Drawing for the job (mm, zero at the part's lowest x, y, z). A direction names the side the tool comes from. Round coordinates to 2 decimals unless told otherwise and drop trailing zeros. Write each loop counter-clockwise with the first axis right and the second up, starting at its lowest first coordinate (ties: lowest second). Pieces come first, ordered by that corner, then holes. Notation, with made-up numbers: M -7,15 L 2,15 A8 ccw 2,25 Z; hole C 60,19.5 d9. An arc over 180 degrees is marked long. Use a Markdown table: item, result.
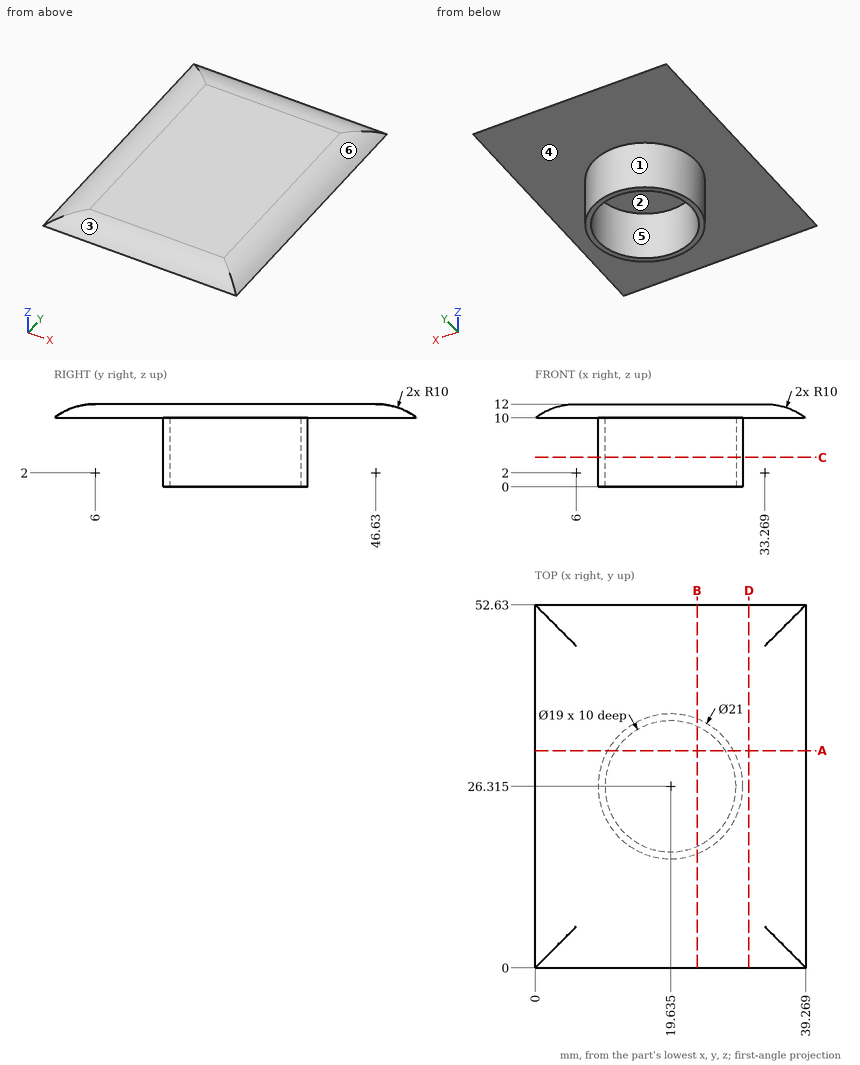
Q1. Which spindle directions (+Z, -Z, +X, -X, +Y, -Y) get a long thin tool onto all of the face, cutting with end or side? Do the marked faces 5 and 6. Say none if no direction does.
Response values:
| item | result |
|---|---|
| face 5 | -Z |
| face 6 | +Z, +X, +Y, -Y |
Q2. Drill centre lines: L1, parallel to X at y = 26, z = 2.25; L2, parallel to Y at x = 21, z = 3.5 (1 decimal); L3, parallel to Z at x = 18, y = 23. Where is each one in solid material? Low to high.
Response values:
| item | result |
|---|---|
| L1 | x = 9.14 to 10.14, 29.13 to 30.13 |
| L2 | y = 15.9 to 16.9, 35.7 to 36.7 |
| L3 | z = 10 to 12 |
Q3. Cut at C-C on z = 4.25. Give the cut face in (x, y) (1 decimal).
Response values:
| item | result |
|---|---|
| outline | C 19.6,26.3 d21; hole C 19.6,26.3 d19 |
Q4. Drop flat-ended pins along their axis: P1, Ø4, axis at y = 23, z = 9, coming from the +X side; P2, Ø11.5, axis at x = 19.63, y = 26.32, coming from the -Z side; P3, Ø1, axis at x = 22, z = 9, coming from the -Y side. Give the stop position or say it passes through.
Response values:
| item | result |
|---|---|
| P1 | stops at x = 39.27 |
| P2 | stops at z = 10 |
| P3 | stops at y = 15.98 |
Q5. Cut at A-A on y = 31.5. Give the cut face in (x, z) (1 decimal).
Response values:
| item | result |
|---|---|
| outline | M 0,10 L 10.5,10 L 10.5,0 L 11.7,0 L 11.7,10 L 27.6,10 L 27.6,0 L 28.8,0 L 28.8,10 L 39.3,10 A10 ccw 33.3,12 L 6,12 A10 ccw Z |
Q6. Cut at D-D on x = 31. Give the cut face in (y, z).
Response values:
| item | result |
|---|---|
| outline | M 0,10 L 52.63,10 A10 ccw 46.63,12 L 6,12 A10 ccw Z |
Q7. Cut at B-B on x = 23.5. Give the cut face in (y, z).
Response values:
| item | result |
|---|---|
| outline | M 0,10 L 16.55,10 L 16.55,0 L 17.64,0 L 17.64,10 L 34.99,10 L 34.99,0 L 36.08,0 L 36.08,10 L 52.63,10 A10 ccw 46.63,12 L 6,12 A10 ccw Z |
Q8. Two-plate mould, pull along Y, no slides. Class the marked faces 1, 2, 3 and 4: +Y half, -Y half, draft (parallel to the pull), parting line (faces both ways), or undercut.
Response values:
| item | result |
|---|---|
| face 1 | parting line |
| face 2 | undercut |
| face 3 | -Y half |
| face 4 | draft |
